from build123d import *

# Parameters (mm, degrees)
SKETCH1_W           = 160
SKETCH1_H           = 150
BOSS_EXTRUDE1_DEPTH = 16
SKETCH2_W           = 14
SKETCH2_H           = 14
CUT_EXTRUDE1_DEPTH  = 14
SKETCH3_R           = 3
CUT_EXTRUDE2_DEPTH  = 220.899977262


with BuildPart() as part:
    # Sketch1 → Boss-Extrude1 (new body)
    with BuildSketch(Plane.XY):
        with Locations((-80, -75)):
            Rectangle(SKETCH1_W, SKETCH1_H)
    extrude(amount=BOSS_EXTRUDE1_DEPTH)

    # Sketch2 → Cut-Extrude1 (cut)
    with BuildSketch(Plane.XY.offset(16)):
        with Locations((-80, -12.5)):
            Rectangle(SKETCH2_W, SKETCH2_H)
        with Locations((-134.126587737, -106.25)):
            Rectangle(SKETCH2_W, SKETCH2_H)
        with Locations((-25.873412263, -106.25)):
            Rectangle(SKETCH2_W, SKETCH2_H)
    extrude(amount=-CUT_EXTRUDE1_DEPTH, mode=Mode.SUBTRACT)

    # Sketch3 → Cut-Extrude2 (cut, through all)
    with BuildSketch(Plane.XY.offset(16)):
        with Locations((-65, -43)):
            Circle(SKETCH3_R)
        with Locations((-150, -43)):
            Circle(SKETCH3_R)
    extrude(amount=-CUT_EXTRUDE2_DEPTH, mode=Mode.SUBTRACT)


solid = part.part
The model under review builds one solid part; all positions refer to its coordinate system, in mm. A direction names the side the tool comes from. Round coordinates to 2 decimals unless told otherwise and drop trailing zeros. Loops run counter-clockwise (first coordinate to the right, second up) from the corner with the lowest first, then second, coordinate; pieces in that order, holes last. Notation, with made-up numbers: (85.25, 26.5) - (136.25, 26.5) arc R12 cw to (136.25, 45.5) - close; hole circle Ø8 at (71.5, 6). An arc over 180 degrees is marked (long way). Use CSV: the item, a comma, the result in double quotes.
(1) The part is to be moulded in two halves that separate along Y. For faces 3 (the flat face through (-32.873, -106, 9)), 4 (the flat face through (-81, -150, 8)), 5 (the flat face through (-160, -76, 8)), say which applies: pulls with the +Y half, pulls with the -Y half, needs draft (parallel to the pull), parting line crosses it, or undercut.
Working result:
face 3,"undercut"
face 4,"pulls with the -Y half"
face 5,"needs draft"
(2) Take a section at B-B, the plane y = -43. Give the boundary of the cut face in (x, z).
Working result:
outline,"(-160, 0) - (-153, 0) - (-153, 16) - (-160, 16) - close; (-147, 0) - (-68, 0) - (-68, 16) - (-147, 16) - close; (-62, 0) - (0, 0) - (0, 16) - (-62, 16) - close"
(3) Take a section at D-D, the plane y = -102. Give the boundary of the cut face in (x, z).
Working result:
outline,"(-160, 0) - (0, 0) - (0, 16) - (-18.87, 16) - (-18.87, 2) - (-32.87, 2) - (-32.87, 16) - (-127.13, 16) - (-127.13, 2) - (-141.13, 2) - (-141.13, 16) - (-160, 16) - close"
(4) Take a section at C-C, the plane z = 9.75. Give the boundary of the cut face in (x, y).
Working result:
outline,"(-160, -150) - (0, -150) - (0, 0) - (-160, 0) - close; hole circle Ø6 at (-150, -43); hole (-141.13, -113.25) - (-127.13, -113.25) - (-127.13, -99.25) - (-141.13, -99.25) - close; hole (-87, -19.5) - (-73, -19.5) - (-73, -5.5) - (-87, -5.5) - close; hole circle Ø6 at (-65, -43); hole (-32.87, -113.25) - (-18.87, -113.25) - (-18.87, -99.25) - (-32.87, -99.25) - close"
(5) For line 1 (Y direction, x = -150, z = 12.75); line 2 (Y direction, x = -127.5, z = 6); line 3 (X direction, y = -17, z = 2.5), list the stretches that pass through material, from the lowest coordinate up.
Working result:
line 1,"y = -150 to -46, -40 to 0"
line 2,"y = -150 to -113.25, -99.25 to 0"
line 3,"x = -160 to -87, -73 to 0"
(6) Take a section at A-A, the plane x = -150. Give the boundary of the cut face in (y, z), plus the area to 3 significant figures.
Working result:
outline,"(-150, 0) - (-46, 0) - (-46, 16) - (-150, 16) - close; (-40, 0) - (0, 0) - (0, 16) - (-40, 16) - close"
area,"2,300 mm^2"
(7) Clearance check with flat-ended pins moving along their axes: P1, Ø4, axis at x = -24, y = -105.5, coming from the +Z side; P2, Ø5, axis at x = -65, y = -43, coming from the +Z side. State where each tip first meets the part, or that it passes through.
Working result:
P1,"stops at z = 2"
P2,"passes through"
(8) Machinability: for faces 1 (the flat face through (0, -76, 8)), 2 (the flat face through (-18.873, -106, 9)), which of the approach directions +Z, -Z, +X, -X, +Y, -Y give a long, thin tool a straight path to every point of the face, cutting with its end or side? Answer none if there is none.
Working result:
face 1,"+Z, -Z, +X, +Y, -Y"
face 2,"+Z"
